```python
from build123d import *

# Parameters (mm, degrees)
BOSS_EXTRUDE1_DEPTH     = 127
SKETCH3_W               = 5
SKETCH3_H               = 42.3
BOSS_EXTRUDE2_DEPTH     = 42.3
SKETCH4_R               = 1.7
CUT_EXTRUDE1_DEPTH      = 5
CUT_EXTRUDE7_DEPTH      = 161.690696682
CUT_EXTRUDE7_DEPTH_BACK = 161.690696682
SKETCH5_R               = 1.7
SKETCH8_R               = 3.2
CUT_EXTRUDE8_DEPTH      = 2
SKETCH10_W              = 20
SKETCH10_H              = 10
BOSS_EXTRUDE3_DEPTH     = 35
FILLET3_R               = 5
SKETCH12_R              = 1.7
CUT_EXTRUDE9_DEPTH      = 35
RIB47_START             = -2
RIB47_DEPTH             = 2
FILLET7_R               = 5
FILLET8_R               = 2
SKETCH18_W              = 6.4
SKETCH18_H              = 20
CUT_EXTRUDE10_DEPTH     = 9
SKETCH19_W              = 5
SKETCH19_H              = 18
CUT_EXTRUDE11_DEPTH     = 4


# Read off the part's stored shape, not the designer's step: Rib47
with BuildPart() as part:
    # Sketch2 → Boss-Extrude1 (new body)
    with BuildSketch(Plane(origin=(0, 0, 0), x_dir=(1, 0, 0), z_dir=(0, 1, 0))):
        with BuildLine():
            ThreePointArc((-4.546695502, 0), (-4.968391225, -0.231350196), (-4.999849396, -0.711309131))
            Line((-4.999849396, -0.711309131), (-3.66337779, -3.577381738))
            ThreePointArc((-3.66337779, -3.577381738), (-3.726294131, -4.537299608), (-4.569685577, -5))
            Line((-4.569685577, -5), (-45.823162248, -5))
            ThreePointArc((-45.823162248, -5), (-46.689187651, -4.5), (-46.689187651, -3.5))
            Line((-46.689187651, -3.5), (-45.101474411, -0.75))
            ThreePointArc((-45.101474411, -0.75), (-45.101474411, -0.25), (-45.534487113, 0))
            Line((-45.534487113, 0), (-54.465512887, 0))
            ThreePointArc((-54.465512887, 0), (-54.898525589, -0.25), (-54.898525589, -0.75))
            Line((-54.898525589, -0.75), (-53.310812349, -3.5))
            ThreePointArc((-53.310812349, -3.5), (-53.310812349, -4.5), (-54.176837752, -5))
            Line((-54.176837752, -5), (-81.4, -5))
            ThreePointArc((-81.4, -5), (-86.703300859, -7.196699141), (-88.9, -12.5))
            Line((-88.9, -12.5), (-88.9, -17.5))
            ThreePointArc((-88.9, -17.5), (-86.703300859, -22.803300859), (-81.4, -25))
            Line((-81.4, -25), (81.4, -25))
            ThreePointArc((81.4, -25), (86.703300859, -22.803300859), (88.9, -17.5))
            Line((88.9, -17.5), (88.9, -12.5))
            ThreePointArc((88.9, -12.5), (86.703300859, -7.196699141), (81.4, -5))
            Line((81.4, -5), (54.176837752, -5))
            ThreePointArc((54.176837752, -5), (53.310812349, -4.5), (53.310812349, -3.5))
            Line((53.310812349, -3.5), (54.898525589, -0.75))
            ThreePointArc((54.898525589, -0.75), (54.898525589, -0.25), (54.465512887, 0))
            Line((54.465512887, 0), (45.534487113, 0))
            ThreePointArc((45.534487113, 0), (45.101474411, -0.25), (45.101474411, -0.75))
            Line((45.101474411, -0.75), (46.689187651, -3.5))
            ThreePointArc((46.689187651, -3.5), (46.689187651, -4.5), (45.823162248, -5))
            Line((45.823162248, -5), (4.569685577, -5))
            ThreePointArc((4.569685577, -5), (3.726294131, -4.537299608), (3.66337779, -3.577381738))
            Line((3.66337779, -3.577381738), (4.999849396, -0.711309131))
            ThreePointArc((4.999849396, -0.711309131), (4.968391225, -0.231350196), (4.546695502, 0))
            Line((4.546695502, 0), (-4.546695502, 0))
        make_face()
    extrude(amount=BOSS_EXTRUDE1_DEPTH)

    # Sketch3 → Boss-Extrude2 (add)
    with BuildSketch(Plane.XY.offset(25)):
        with Locations((-13.06, 55.018873206)):
            Rectangle(SKETCH3_W, SKETCH3_H)
    extrude(amount=BOSS_EXTRUDE2_DEPTH)

    # Sketch4 → Cut-Extrude1 (cut)
    with BuildSketch(Plane(origin=(-10.56, 0, 0), x_dir=(0, 0, -1), z_dir=(1, 0, 0))):
        with BuildLine():
            ThreePointArc((-34.95, 55.018873206), (-46.15, 66.218873206), (-57.35, 55.018873206))
            Line((-57.35, 55.018873206), (-34.95, 55.018873206))
        make_face()
        with BuildLine():
            Line((-34.95, 55.018873206), (-57.35, 55.018873206))
            ThreePointArc((-57.35, 55.018873206), (-46.15, 43.818873206), (-34.95, 55.018873206))
        make_face()
        with Locations((-61.65, 70.518873206)):
            Circle(SKETCH4_R)
        with Locations((-30.65, 70.518873206)):
            Circle(SKETCH4_R)
        with Locations((-30.65, 39.518873206)):
            Circle(SKETCH4_R)
        with Locations((-61.65, 39.518873206)):
            Circle(SKETCH4_R)
    extrude(amount=-CUT_EXTRUDE1_DEPTH, mode=Mode.SUBTRACT)

    # Sketch5 → Cut-Extrude7 (cut, two sides: drawn at the far end of the back side and taken through both)
    with BuildSketch(Plane.XY.offset(25).offset(-CUT_EXTRUDE7_DEPTH_BACK)):
        with Locations((-58.65, 118.5)):
            Circle(SKETCH5_R)
        with Locations(Location((58.65, 118.5, 0), (0, 0, 180))):
            Circle(SKETCH5_R)
        with Locations(Location((58.65, 8.5, 0), (0, 0, 180))):
            Circle(SKETCH5_R)
        with Locations((-58.65, 8.5)):
            Circle(SKETCH5_R)
    extrude(amount=CUT_EXTRUDE7_DEPTH + CUT_EXTRUDE7_DEPTH_BACK, mode=Mode.SUBTRACT)

    # Sketch8 → Cut-Extrude8 (cut)
    with BuildSketch(Plane(origin=(0, 0, 5), x_dir=(-1, 0, 0), z_dir=(0, 0, -1))):
        with Locations((-58.65, 118.5)):
            Circle(SKETCH8_R)
        with Locations((-58.65, 8.5)):
            Circle(SKETCH8_R)
        with Locations((58.65, 118.5)):
            Circle(SKETCH8_R)
        with Locations((58.65, 8.5)):
            Circle(SKETCH8_R)
    extrude(amount=-CUT_EXTRUDE8_DEPTH, mode=Mode.SUBTRACT)

    # Sketch10 → Boss-Extrude3 (add)
    with BuildSketch(Plane.XY.offset(25)):
        with Locations((0, 5)):
            Rectangle(SKETCH10_W, SKETCH10_H)
    extrude(amount=BOSS_EXTRUDE3_DEPTH)

    # Fillet3
    fillet3_edges = [part.edges().sort_by_distance(p)[0] for p in [
        (-10, 5, 60),
        (10, 5, 60),
    ]]
    fillet(fillet3_edges, radius=FILLET3_R)

    # Sketch12 → Cut-Extrude9 (cut)
    with BuildSketch(Plane(origin=(0, 10, 0), x_dir=(1, 0, 0), z_dir=(0, 1, 0))):
        with Locations(Location((0, -54, 0), (0, 0, 270))):
            Circle(SKETCH12_R)
    extrude(amount=-CUT_EXTRUDE9_DEPTH, mode=Mode.SUBTRACT)

    # Rib47 outline → Rib47 (add)
    with BuildSketch(Plane(origin=(10, 0, 0), x_dir=(0, 0, -1), z_dir=(1, 0, 0)).offset(RIB47_START)):
        Polygon((-25, 35.191123447), (-50.191123447, 10), (-25, 10), align=None)
    rib47 = extrude(amount=RIB47_DEPTH)

    # Mirror1: Rib47 across plane
    add(rib47.mirror(Plane(origin=(0, 0, 0), x_dir=(0, 0, 1), z_dir=(1, 0, 0))))

    # Fillet7
    # the kernel refuses this fillet: 5 mm, written as the material it adds along each edge
    with BuildSketch(Plane(origin=(-10, 47.691123447, 25), x_dir=(-1, 0, 0), z_dir=(0, -1, 0))) as fillet7_piece_1_section:
        with BuildLine():
            CenterArc((FILLET7_R, -FILLET7_R), FILLET7_R, 90, 90)
            Line((0, -FILLET7_R), (0, 0))
            Line((0, 0), (FILLET7_R, 0))
        make_face()
    fillet7_piece_1 = extrude(amount=47.691123447, mode=Mode.PRIVATE)
    fillet7_piece_1 = split(fillet7_piece_1, bisect_by=Plane(origin=(-11.152129269, 25.569946894, 34.621176553), z_dir=(0, -0.7071067811865476, -0.7071067811865476)), keep=Keep.TOP, mode=Mode.PRIVATE)
    add(fillet7_piece_1)
    with BuildSketch(Plane(origin=(10, 47.691123447, 25), x_dir=(0, 0, 1), z_dir=(0, -1, 0))) as fillet7_piece_2_section:
        with BuildLine():
            CenterArc((FILLET7_R, -FILLET7_R), FILLET7_R, 90, 90)
            Line((0, -FILLET7_R), (0, 0))
            Line((0, 0), (FILLET7_R, 0))
        make_face()
    fillet7_piece_2 = extrude(amount=47.691123447, mode=Mode.PRIVATE)
    fillet7_piece_2 = split(fillet7_piece_2, bisect_by=Plane(origin=(11.152129269, 25.569946894, 34.621176553), z_dir=(0, -0.7071067811865476, -0.7071067811865476)), keep=Keep.TOP, mode=Mode.PRIVATE)
    add(fillet7_piece_2)

    # Fillet8
    fillet8_edges = [part.edges().sort_by_distance(p)[0] for p in [
        (0, 10, 25),
        (8, 22.595561724, 25),
        (11.5, 35.191123447, 25),
        (-9.28, 35.191123447, 25),
        (-8, 22.595561724, 25),
    ]]
    fillet(fillet8_edges, radius=FILLET8_R)

    # Sketch18 → Cut-Extrude10 (cut)
    with BuildSketch(Plane(origin=(0, 10, 0), x_dir=(1, 0, 0), z_dir=(0, 1, 0))):
        with Locations((0, -39.517084206)):
            Rectangle(SKETCH18_W, SKETCH18_H)
    extrude(amount=-CUT_EXTRUDE10_DEPTH, mode=Mode.SUBTRACT)

    # Sketch19 → Cut-Extrude11 (cut)
    with BuildSketch(Plane(origin=(0, 1, 0), x_dir=(1, 0, 0), z_dir=(0, 1, 0))):
        with Locations((0, -40.017084206)):
            Rectangle(SKETCH19_W, SKETCH19_H)
    extrude(amount=-CUT_EXTRUDE11_DEPTH, mode=Mode.SUBTRACT)


solid = part.part
```
The model under review builds one solid part; all positions refer to its coordinate system, in mm. A direction names the side the tool comes from. Round coordinates to 2 decimals unless told otherwise and drop trailing zeros. Order: outer loops, then holes, each group sorted by start corner. A loop starts at its lowest first (then second) coordinate and runs counter-clockwise, first axis right, second up.
Item 1: For pin 1 (4 mm diameter, centred on x = -13, z = 37.5, fed in from -Y); pin 2 (7.5 mm diameter, centred on y = 15.5, z = 39.5, fed in from +X); pin 3 (1.5 mm diameter, centred on x = 59, y = 95.5, fed in from -Z), all flat-tipped, find the tip position at first contact; note any pin that passes through.
Working result:
pin 1: stops at y = 33.87
pin 2: stops at x = 10
pin 3: stops at z = 5
Item 2: Draft analysis for pull direction Y (two halves, no side actions). For faces 6 (the cylindrical face through (-56.29, 120.66, 5.99)), 7 (the flat face through (68, 63, 5)), 8 (the flat face through (-13, 76.169, 46)), state which applies: released by +Y, released by -Y, zero draft, split by the parting line, or undercut.
Working result:
face 6: undercut
face 7: zero draft
face 8: released by +Y
Item 3: To check wall thickness, follow probe 1 along X at (y, z) = (118.5, 15.5); probe 2 along Y at (x, z) = (-58.65, 14); probe 3 along Y at (x, z) = (-58.65, 5.8). State the ranges of each line that lie inside material, in increasing order.
Working result:
probe 1: x = -88.9 to -60.35, -56.95 to 56.95, 60.35 to 88.9
probe 2: y = 0 to 6.8, 10.2 to 116.8, 120.2 to 127
probe 3: y = 0 to 5.3, 11.7 to 115.3, 121.7 to 127
Item 4: Add section C-C, the plane x = -42.5. State the section outline as (y, z) points.
Working result:
outline: (0, 5) - (127, 5) - (127, 25) - (0, 25) - close
Item 5: Add section B-B, the plane z = 40. State the section outline as (x, y) points.
Working result:
outline: (-15.56, 33.87) - (-10.56, 33.87) - (-10.56, 45.66) - (-15.56, 45.66) - close; (-15.56, 64.38) - (-10.56, 64.38) - (-10.56, 76.17) - (-15.56, 76.17) - close; (-10, 0) - (-2.5, 0) - (-2.5, 1) - (-3.2, 1) - (-3.2, 10) - (-8, 10) - (-8, 20.19) - (-10, 20.19) - close; (2.5, 0) - (10, 0) - (10, 20.19) - (8, 20.19) - (8, 10) - (3.2, 10) - (3.2, 1) - (2.5, 1) - close
Item 6: Machinability: for faces 1 (the flat face through (-60, 7, 7)), 2 (the flat face through (3.2, 6, 40)), 3 (the flat face through (-10.56, 64, 55)), 4 (the flat face through (8, 17, 34)), 5 (the cylindrical face through (-13.02, 61.83, 37.26)), which of the approach directions +Z, -Z, +X, -X, +Y, -Y give a long, thin tool a straight path to every point of the face, cutting with its end or side? Answer none if there is none.
Working result:
face 1: -Z
face 2: +Y
face 3: +Z, +X, +Y
face 4: +Z, +Y
face 5: +X, -X
